For this review, take the finished solid that the model builds, in its own axes (mm). A direction names the side the tool comes from. Round coordinates to 2 decimals unless told otherwise and drop trailing zeros. Loops run counter-clockwise (first coordinate to the right, second up) from the corner with the lowest first, then second, coordinate; pieces in that order, holes last. Notation, with made-up numbers: M 44.5,70 L 77.5,70 A32 ccw 77.5,109 Z; hole C 78.5,-19 d4. An arc over 180 degrees is marked long. One line per question, with ' | ' between items. Start each with the question number.
1) We need section D-D (x = 22.5). Give the boundary of the cut face in (y, z), and give its area (3 significant figures).
2) For probe 1 along Y at (x, z) = (0, 5.5); probe 2 along Y at (x, z) = (0, 11.25); probe 3 along Z at (x, y) = (0, 99), list the stretches that pass through material, from the lowest coordinate up. Write a range as from..to.
3) For faces 4 (the face through (0, 17.5, 17)), 5 (the face through (-0.385, -17.496, 12.325)), 6 (the face through (-17.5, 4, 12)), 7 (the face through (0.1, 17.5, 6.9)), 8 (the face through (-36, 22.5, 7)), list the 3-axis set-ups (+Z, -Z, +X, -X, +Y, -Y) from which the entire face can be reached by the end or side of a thin tool; tool diameter is ignored.
4) We need section B-B (z = 12.75). Give the boundary of the cut face in (x, y).
5) Mouldability with a two-part tool opening along X and no side actions: class faces 1 (the face through (-56.486, 102.797, 4.93)), 2 (the face through (-52.99, 99.22, 7.46)), 3 (the face through (0, 107, 10)) as pulls with the +X half, pulls with the -X half, needs draft (parallel to the pull), parting line crosses it, or undercut.
6) For pin 1 Ø6 at (y, z) = (4.5, 10.5) entering from +X; pin 2 Ø5 at (y, z) = (1.5, 18) entering from -X; pin 3 Ø8 at (x, z) = (38.5, 3) entering from -Y, all flat-tipped, find the tip position at first contact; note any pin that passes through.
7) We need section C-C (y = 28). Give the boundary of the cut face in (x, z).
8) We need section A-A (z = 22.5). Give the boundary of the cut face in (x, y), and give its area (3 significant figures).
```python
from build123d import *

# Parameters (mm, degrees)
F0_R         = 12.5
F1_DEPTH     = 10
F2_R         = 12.5
F3_DEPTH     = 15
F4_T         = 5
F4_T3_DEPTH  = 20
F5_R         = 10
F6_T1_DEPTH  = 40
F7_T1_DEPTH  = 5
F7_T6_DEPTH  = 92.3194198861
F7_T13_DEPTH = 48.659709943


# Not quite as in the source:
# - a fillet or chamfer that OpenCascade refuses, or shapes differently, is made with other operations: its cross-section is extruded or revolved along the edge and cut away or added
# - a shell that OpenCascade refuses in one call is made with other operations: the cavity is built on its own and cut out


with BuildPart() as f1:
    # F0 (on Top) → F1 (new body)
    with BuildSketch(Plane.XY):
        with BuildLine():
            Line((17.5, 0), (17.5, 17.5))
            Line((17.5, 17.5), (0, 17.5))
            ThreePointArc((0, 17.5), (12.3743686708, 12.3743686708), (17.5, 0))
        make_face()
        with BuildLine():
            Line((0, 17.5), (-17.5, 17.5))
            Line((-17.5, 17.5), (-17.5, 0))
            ThreePointArc((-17.5, 0), (-12.3743686708, 12.3743686708), (0, 17.5))
        make_face()
        with BuildLine():
            ThreePointArc((17.5, 0), (12.3743686708, 12.3743686708), (0, 17.5))
            ThreePointArc((0, 17.5), (-12.3743686708, 12.3743686708), (-17.5, 0))
            ThreePointArc((-17.5, 0), (0, -17.5), (17.5, 0))
        make_face()
        Circle(F0_R, mode=Mode.SUBTRACT)
        with BuildLine():
            Line((42.5, 108.5), (0, 108.5))
            Line((0, 108.5), (-42.5, 108.5))
            ThreePointArc((-42.5, 108.5), (-56.6421356237, 102.6421356237), (-62.5, 88.5))
            Line((-62.5, 88.5), (-62.5, 37.5))
            ThreePointArc((-62.5, 37.5), (-56.6421356237, 23.3578643763), (-42.5, 17.5))
            Line((-42.5, 17.5), (-17.5, 17.5))
            Line((-17.5, 17.5), (0, 17.5))
            Line((0, 17.5), (17.5, 17.5))
            Line((17.5, 17.5), (42.5, 17.5))
            ThreePointArc((42.5, 17.5), (56.6421356237, 23.3578643763), (62.5, 37.5))
            Line((62.5, 37.5), (62.5, 88.5))
            ThreePointArc((62.5, 88.5), (56.6421356237, 102.6421356237), (42.5, 108.5))
        make_face()
    extrude(amount=F1_DEPTH)

    # F2 (on face) → F3 (join)
    with BuildSketch(Plane.XY.offset(10)):
        with BuildLine():
            Line((17.5, 17.5), (-17.5, 17.5))
            Line((-17.5, 17.5), (-17.5, 0))
            ThreePointArc((-17.5, 0), (0, -17.5), (17.5, 0))
            Line((17.5, 0), (17.5, 17.5))
        make_face()
        Circle(F2_R, mode=Mode.SUBTRACT)
    extrude(amount=F3_DEPTH)

    # F4: shell of thickness 5, made by hand


with BuildPart() as f4_core1:
    # F4_t2: copy of F1
    add(f1.part)

    # the walls: a layer under each face that stays
    f4_faces = [f4_core1.faces().sort_by_distance(p)[0] for p in [
        (0, -17.5, 12.5),
        (0, 45.5, 0),
        (-12.5, 0, 12.5),
        (-30, 17.5, 5),
        (0, 17.5, 17.5),
        (-56.6421356237, 23.3578643763, 5),
        (-62.5, 63, 5),
        (-56.6421356237, 102.6421356237, 5),
        (0, 108.5, 5),
        (56.6421356237, 102.6421356237, 5),
        (62.5, 63, 5),
        (56.6421356237, 23.3578643763, 5),
        (30, 17.5, 5),
        (17.5, 8.75, 12.5),
        (-11.6666666667, -11.6666666667, 25),
        (-17.5, 8.75, 12.5),
    ]]
    thicken(f4_faces, amount=-F4_T, mode=Mode.SUBTRACT)

    # F4_s4 → F4_t3 (cut)
    with BuildSketch(Plane.XY.offset(-5)):
        Polygon((-17.55, 17.45), (-17.5, 22.5), (-12.5, 22.5), (-12.5, 17.5), align=None)
        Polygon((17.55, 17.45), (17.5, 22.5), (12.5, 22.5), (12.5, 17.5), align=None)
    extrude(amount=F4_T3_DEPTH, mode=Mode.SUBTRACT)


with BuildPart() as f1_1:
    add(f1.part)

    # what is left inside the walls is the cavity
    f4_cavity = [f4_core1.part.solids().sort_by_distance(p)[0] for p in [
        (0, 42.664966, 5.05),
    ]]
    add(f4_cavity, mode=Mode.SUBTRACT)

    # F5
    f5_edges = [f1_1.edges().sort_by_distance(p)[0] for p in [
        (17.5, 17.5, 5),
        (-17.5, 17.5, 5),
    ]]
    fillet(f5_edges, radius=F5_R)

    # F6: fillet of radius 10 on 2 edges, made by hand

    # F6_s2 → F6_t1 (cut)
    with BuildSketch(Plane.XY.offset(10)):
        with BuildLine():
            ThreePointArc((7.5, 17.5), (14.5710678119, 14.5710678119), (17.5, 7.5))
            Line((17.5, 7.5), (17.5, 17.5))
            Line((17.5, 17.5), (7.5, 17.5))
        make_face()
        with BuildLine():
            ThreePointArc((-17.5, 7.5), (-14.5710678119, 14.5710678119), (-7.5, 17.5))
            Line((-7.5, 17.5), (-17.5, 17.5))
            Line((-17.5, 17.5), (-17.5, 7.5))
        make_face()
    extrude(amount=F6_T1_DEPTH, mode=Mode.SUBTRACT)

    # F7: fillet of radius 20 on 2 edges, made by hand

    # F7_s2 → F7_t1 (cut)
    with BuildSketch(Plane.XY.offset(5)):
        with BuildLine():
            ThreePointArc((12.5, 12.2474487139), (19.8383956996, 19.7474487139), (29.9638839772, 22.5))
            Line((29.9638839772, 22.5), (12.5, 22.5))
            Line((12.5, 22.5), (12.5, 12.2474487139))
        make_face()
        with BuildLine():
            ThreePointArc((-29.9638839772, 22.5), (-19.8383956996, 19.7474487139), (-12.5, 12.2474487139))
            Line((-12.5, 12.2474487139), (-12.5, 22.5))
            Line((-12.5, 22.5), (-29.9638839772, 22.5))
        make_face()
    extrude(amount=F7_T1_DEPTH, mode=Mode.SUBTRACT)


with BuildPart() as f7_tool4:
    # F7_s5 → F7_t6 (new body)
    with BuildSketch(Plane.XY.offset(-38.659709943)):
        with BuildLine():
            ThreePointArc((12.5, 12.2474487139), (19.8383956996, 19.7474487139), (29.9638839772, 22.5))
            Line((29.9638839772, 22.5), (12.5, 22.5))
            Line((12.5, 22.5), (12.5, 12.2474487139))
        make_face()
    extrude(amount=F7_T6_DEPTH)

    split(bisect_by=Plane.XZ.offset(-12.5), keep=Keep.TOP)

    split(bisect_by=Plane.XY.offset(20), keep=Keep.BOTTOM)

    split(bisect_by=Plane.XY.offset(10), keep=Keep.TOP)


with BuildPart() as f1_2:
    add(f1_1.part)

    # F7_t3: cut F7_tool4
    add(f7_tool4.part, mode=Mode.SUBTRACT)


with BuildPart() as f7_tool11:
    # F7_s12 → F7_t13 (new body)
    with BuildSketch(Plane.XY.offset(5)):
        with BuildLine():
            ThreePointArc((-29.9638839772, 22.5), (-19.8383956996, 19.7474487139), (-12.5, 12.2474487139))
            Line((-12.5, 12.2474487139), (-12.5, 22.5))
            Line((-12.5, 22.5), (-29.9638839772, 22.5))
        make_face()
    extrude(amount=F7_T13_DEPTH)

    split(bisect_by=Plane.XZ.offset(-12.5), keep=Keep.TOP)

    split(bisect_by=Plane.XY.offset(20), keep=Keep.BOTTOM)


with BuildPart() as f1_3:
    add(f1_2.part)

    # F7_t10: cut F7_tool11
    add(f7_tool11.part, mode=Mode.SUBTRACT)


solid = f1_3.part
```
Answers below:
1) outline: M 16.16,0 L 108.5,0 L 108.5,10 L 103.5,10 L 103.5,5 L 21.06,5 L 21.06,10 L 16.16,10 Z | area: 511 mm^2
2) probe 1: -17.5..-12.5, 12.5..17.5, 103.5..108.5 | probe 2: -17.5..-12.5, 12.5..17.5 | probe 3: 0..5
3) face 4: +Z, +X, -X, +Y | face 5: +Z, -Z, -Y | face 6: +Z, -Z, -X, -Y | face 7: none | face 8: +Z
4) outline: M -17.5,0 A17.5 ccw 17.5,0 L 17.5,7.5 A10 ccw 7.5,17.5 L -7.5,17.5 A10 ccw -17.5,7.5 Z; hole M -12.64,12.5 A20 cw -12.5,12.25 A17.5 cw -12.25,12.5 Z; hole C 0,0 d25; hole M 12.25,12.5 A17.5 cw 12.5,12.25 A20 cw 12.64,12.5 Z
5) face 1: pulls with the -X half | face 2: undercut | face 3: needs draft
6) pin 1: x = 17.5 | pin 2: x = -17.5 | pin 3: y = 17.5
7) outline: M -60.1,0 L 60.1,0 L 60.1,10 L 54.11,10 L 54.11,5 L -54.11,5 L -54.11,10 L -60.1,10 Z
8) outline: M -17.5,0 A17.5 ccw 17.5,0 L 17.5,7.5 A10 ccw 7.5,17.5 L -7.5,17.5 A10 ccw -17.5,7.5 Z; hole C 0,0 d25 | area: 560 mm^2
